Geometry: final body of the model. Coordinates: model frame, mm. A direction names the side the tool comes from. Round coordinates to 2 decimals unless told otherwise and drop trailing zeros. Loops run counter-clockwise (first coordinate to the right, second up) from the corner with the lowest first, then second, coordinate; pieces in that order, holes last. Notation, with made-up numbers: (86.25, 13.25) -> (145.25, 13.25) arc R16 ccw to (145.25, 31.25) -> close; hole circle Ø5 at (74.5, 55). An arc over 180 degrees is marked (long way). Answer in a Markdown table with one row per item.
```python
from build123d import *

# Parameters (mm, degrees)
SKETCH1_R           = 5.0254
SKETCH1_R_2         = 9.525
BOSS_EXTRUDE1_DEPTH = 4.445
SKETCH3_R           = 5.715
CUT_EXTRUDE4_DEPTH  = 238.309326519
SKETCH2_R           = 6.4135
BOSS_EXTRUDE2_DEPTH = 4.445
SKETCH6_W           = 13.50293176
SKETCH6_H           = 6.21934711
CUT_EXTRUDE6_DEPTH  = 2.54


with BuildPart() as part:
    # Sketch1 → Boss-Extrude1 (new body)
    with BuildSketch(Plane.XY):
        with BuildLine():
            Line((-17.211015945, 18.751241343), (43.963752379, 74.901119305))
            ThreePointArc((43.963752379, 74.901119305), (214.381413502, 0), (43.963752379, -74.901119305))
            Line((43.963752379, -74.901119305), (-17.211015945, -18.751241343))
            ThreePointArc((-17.211015945, -18.751241343), (-25.452467891, 0), (-17.211015945, 18.751241343))
        make_face()
        Circle(SKETCH1_R, mode=Mode.SUBTRACT)
        with Locations((112.7125, 0)):
            Circle(SKETCH1_R_2, mode=Mode.SUBTRACT)
    extrude(amount=BOSS_EXTRUDE1_DEPTH)

    # Sketch3 → Cut-Extrude4 (cut, through all)
    with BuildSketch(Plane.XY):
        with Locations((49.363448016, -28.5)):
            Circle(SKETCH3_R)
    extrude(amount=CUT_EXTRUDE4_DEPTH, mode=Mode.SUBTRACT)

    # Sketch2 → Boss-Extrude2 (add)
    with BuildSketch(Plane.XY):
        with BuildLine():
            Line((-24.995388267, 4.801946178), (-37.855905828, -62.140417979))
            ThreePointArc((-37.855905828, -62.140417979), (-28.163364792, -97.115789925), (5.538841954, -110.583650001))
            Line((5.538841954, -110.583650001), (120.834104773, -101.344005785))
            ThreePointArc((120.834104773, -101.344005785), (79.641074663, -96.139735796), (43.963752379, -74.901119305))
            Line((43.963752379, -74.901119305), (-17.211015945, -18.751241343))
            ThreePointArc((-17.211015945, -18.751241343), (-24.166780914, -7.987166081), (-24.995388267, 4.801946178))
        make_face()
        with Locations((2.274488984, -69.85)):
            Circle(SKETCH2_R, mode=Mode.SUBTRACT)
    extrude(amount=BOSS_EXTRUDE2_DEPTH)

    # Sketch6 → Cut-Extrude6 (cut)
    with BuildSketch(Plane(origin=(0, 0, 0), x_dir=(-1, 0, 0), z_dir=(0, 0, -1))):
        with Locations((-95.255563191, 46.998761557)):
            Rectangle(SKETCH6_W, SKETCH6_H)
    extrude(amount=-CUT_EXTRUDE6_DEPTH, mode=Mode.SUBTRACT)


solid = part.part
```
Item 1: Line query: probe 1 along Y at (x, z) = (0, 2.95); probe 2 along X at (y, z) = (48, 0.85); probe 3 along Y at (x, z) = (114.5, 2.8). Output: solid intervals per line, ascending. Write a range as [from, to].
Answer:
| item | result |
|---|---|
| probe 1 | y = [-110.65, -75.85], [-63.85, -5.03], [5.03, 34.55] |
| probe 2 | x = [14.66, 88.5], [102.01, 202.34] |
| probe 3 | y = [-101.85, -9.36], [9.36, 101.65] |
Item 2: Reachability of faces 4 (the face through (121.8, 2.86, 2.19)), 5 (the face through (95, 47, 2.54)) from +Z, -Z, +X, -X, +Y, -Y: full face, straight path, thin tool, end or side. Return the list, or none.
Answer:
| item | result |
|---|---|
| face 4 | +Z, -Z |
| face 5 | -Z |
Item 3: Draft query along Y for faces 1 (the face through (-31.336, -28.201, 2.191)), 2 (the face through (4.793, 1.509, 2.191)), 3 (the face through (86, -3, 0)). Return one class per face: pulls with the +Y half, pulls with the -Y half, needs draft (parallel to the pull), parting line crosses it, or undercut.
Answer:
| item | result |
|---|---|
| face 1 | pulls with the +Y half |
| face 2 | undercut |
| face 3 | needs draft |
Item 4: Cut plane B-B (x = 0). Output: boundary loops of the cut face in (y, z) (3 decimals).
Answer:
| item | result |
|---|---|
| outline | (-110.651, 0) -> (-75.847, 0) -> (-75.847, 4.445) -> (-110.651, 4.445) -> close; (-63.853, 0) -> (-5.025, 0) -> (-5.025, 4.445) -> (-63.853, 4.445) -> close; (5.025, 0) -> (34.549, 0) -> (34.549, 4.445) -> (5.025, 4.445) -> close |
Item 5: Pin query (flat end, axial travel): pin 1 Ø6 at (x, y) = (24, 64.5) entering from +Z; pin 2 Ø1.5 at (y, z) = (-24.5, 2) entering from +X; pin 3 Ø2 at (x, z) = (104.5, 3) entering from +Y; pin 4 Ø1.3 at (x, z) = (97.5, 1.5) entering from +Y. Return the tip coordinate at first contact, or that it passes through.
Answer:
| item | result |
|---|---|
| pin 1 | passes through |
| pin 2 | stops at x = 211.57 |
| pin 3 | stops at y = 101.41 |
| pin 4 | stops at y = 100.62 |
Item 6: Cut plane A-A (z = 1.45). Count the separate pieces of the cut face and the enclosed holes in it, then the cut area to 3 significant figures.
Answer:
| item | result |
|---|---|
| separate pieces | 1 |
| enclosed holes | 5 |
| area | 40,400 mm² |
Item 7: Cut plane C-C (y = -28.5). Output: boundary loops of the cut face in (x, z) (3 decimals).
Answer:
| item | result |
|---|---|
| outline | (-31.393, 0) -> (43.648, 0) -> (43.648, 4.445) -> (-31.393, 4.445) -> close; (55.078, 0) -> (210.305, 0) -> (210.305, 4.445) -> (55.078, 4.445) -> close |
Item 8: Cut plane D-D (x = 51). Output: boundary loops of the cut face in (y, z) (3 decimals).
Answer:
| item | result |
|---|---|
| outline | (-106.94, 0) -> (-33.976, 0) -> (-33.976, 4.445) -> (-106.94, 4.445) -> close; (-23.024, 0) -> (80.797, 0) -> (80.797, 4.445) -> (-23.024, 4.445) -> close |
